Autodesk Inventor part; units mm, degrees
ref_plane "YZ Plane" through (0, 0, 0) normal (1, 0, 0) x (0, 1, 0)
ref_plane "XZ Plane" through (0, 0, 0) normal (0, 1, 0) x (-1, 0, 0)
ref_plane "XY Plane" through (0, 0, 0) normal (0, 0, 1) x (1, 0, 0)
sketch "スケッチ1" plane through (0, 0, 0) normal (0, 1, 0) x (-1, 0, 0)
  circle A0 centre (0, 0) radius 125
  dimension "d0" = 250
sketch "スケッチ2" plane through (0, 0, 0) normal (0, 1, 0) x (-1, 0, 0)
  circle A0 centre (108, 17.5) radius 1.6
  circle A1 centre (108, -17.5) radius 1.6
  circle A2 centre (-38.8446, 102.2807) radius 1.6
  circle A3 centre (-69.1554, 84.7807) radius 1.6
  circle A4 centre (-69.1554, -84.7807) radius 1.6
  circle A5 centre (-38.8446, -102.2807) radius 1.6
  point P0 (0, 0)
  dimension "d5" = 3.2
  dimension "d6" = 3.2
  dimension "d11" = 35
  dimension "d16" = 360
  dimension "d22" = 108
  dimension "d23" = 108
  dimension "d28" = 17.5
extrude "押し出し5" add sketch "スケッチ1" against normal blind 6
extrude "押し出し6" cut sketch "スケッチ2" against normal blind 6
sketch "スケッチ4" plane through (0, 0, 0) normal (0, 1, 0) x (1, 0, 0)
  circle A0 centre (0, 0) radius 116.86
  line L0 (0, 0) -> (-58.43, 101.2037)
  line L1 (0, 0) -> (116.86, 0) construction
  line L2 (0, 0) -> (-58.43, -101.2037)
  line L3 (0, 0) -> (116.86, 0) construction
  line L4 (0, 0) -> (116.86, 0)
  dimension "d33" = 233.72
  dimension "d34" = 120
  dimension "d35" = 120
hole "穴1" at (-58.43, 0, -101.2037) at (-58.43, 0, 101.2037) at (116.86, 0, 0) direction (0, -1, 0) diameter 3.2 depth 10
sketch "スケッチ5" plane through (0, 0, 0) normal (0, 1, 0) x (1, 0, 0)
  circle A0 centre (116.86, 0) radius 1.6
  line L0 (116.86, 0) -> (116.86, 10)
  line L1 (116.86, 0) -> (126.86, 0) construction
  line L2 (116.86, 10) -> (116.86, -10)
  point P0 (0, 0)
  point P1 (-67.0903, 96.2037)
  point P2 (-49.7697, 106.2037)
  point P3 (-49.7697, -106.2037)
  point P4 (-67.0903, -96.2037)
  dimension "d43" = 10
  dimension "d44" = 90
  dimension "d45" = 20
  dimension "d48" = 360
hole "穴2" at (116.86, 0, -10) at (116.86, 0, 10) at (-67.0903, 0, -96.2037) at (-49.7697, 0, -106.2037) at (-49.7697, 0, 106.2037) at (-67.0903, 0, 96.2037) direction (0, -1, 0) diameter 3.2 depth 10
sketch "スケッチ6" plane through (0, 0, 0) normal (0, 1, 0) x (1, 0, 0)
  circle A0 centre (0, 0) radius 15
  dimension "d57" = 30
extrude "押し出し7" cut sketch "スケッチ6" against normal blind 10
properties part number "底板"
Can you work these out from the model? Positions are in its coordinate system, mm. Round coordinates to 2 decimals unless told otherwise and drop trailing zeros. Loops run counter-clockwise (first coordinate to the right, second up) from the corner with the lowest first, then second, coordinate; pieces in that order, holes last.
Item 1: If we mould it in two halves opening along Z, with no side actions, what happens to faces 1 (the cylindrical face through (124.88, -2.96, 5.5)), 2 (the flat face through (2, 0, -26)), 3 (the cylindrical face through (-14.985, -2.958, -0.66))? For each: +Z half, -Z half, draft (parallel to the pull), parting line (faces both ways), or undercut.
Item 2: Suppose I cut it at C-C, the plane z = 34. Write out the boundary of the cut face in (x, y), then the cut area to 3 significant figures.
Item 3: Will these pins go through, and if not, where does the flat tip stop? pin 1 Ø1.9 at (x, z) = (38.84, 102.28) entering from +Y; pin 2 Ø3 at (x, y) = (-94.5, -2) entering from +Z.
Item 4: Suppose I cut it at D-D, the plane x = 104.5. Write out the boundary of the cut face in (y, z).
Item 5: Suppose I cut it at B-B, the plane y = -1.95. State how many separate pieces and enclosed holes the cut face has, then the cut area to 3 significant figures.
Item 6: Please list where these lines run through material, in increasing order: L1, parallel to X at y = -3.85, z = 10; L2, parallel to X at y = -3, z = -4; L3, parallel to Z at x = -1.5, y = -5.15.
Item 7: Suppose I cut it at A-A, the plane x = -5. Write out the boundary of the cut face in (y, z).
Reported:
1. face 1: parting line
1. face 2: draft
1. face 3: undercut
2. outline: (-120.29, -6) - (120.29, -6) - (120.29, 0) - (-120.29, 0) - close
2. area: 1,440 mm2
3. pin 1: passes through
3. pin 2: stops at z = 83.52
4. outline: (-6, -68.59) - (0, -68.59) - (0, 68.59) - (-6, 68.59) - close
5. separate pieces: 1
5. enclosed holes: 16
5. area: 48,300 mm2
6. L1: x = -124.6 to -11.18, 11.18 to 115.26, 118.46 to 124.6
6. L2: x = -124.94 to -14.46, 14.46 to 124.94
6. L3: z = -124.99 to -14.92, 14.92 to 124.99
7. outline: (-6, -124.9) - (0, -124.9) - (0, -14.14) - (-6, -14.14) - close; (-6, 14.14) - (0, 14.14) - (0, 124.9) - (-6, 124.9) - close
